Model file for the job. Use its own axes, mm. Round coordinates to 2 decimals unless told otherwise and drop trailing zeros. Write each loop counter-clockwise with the first axis right and the second up, starting at its lowest first coordinate (ties: lowest second). Pieces come first, ordered by that corner, then holes.
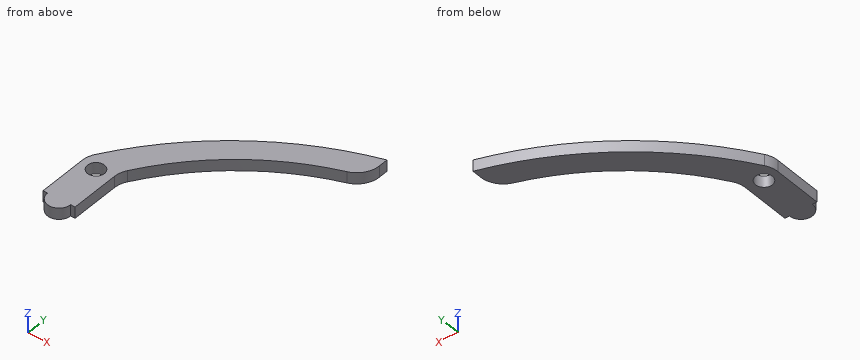
Autodesk Inventor part; units mm, degrees
ref_plane "YZ Plane" through (0, 0, 0) normal (1, 0, 0) x (0, 1, 0)
ref_plane "XZ Plane" through (0, 0, 0) normal (0, 1, 0) x (-1, 0, 0)
ref_plane "XY Plane" through (0, 0, 0) normal (0, 0, 1) x (1, 0, 0)
sketch "Sketch1" plane through (0, 0, 0) normal (0, 0, 1) x (1, 0, 0)
  circle A0 centre (-0.0549, 4.1489) radius 0.75
  line L0 (-1.4285, -0.0001) -> (-1.4285, 4.899)
  line L1 (-1.4285, 4.899) -> (1.4285, 4.899) construction
  line L2 (1.4285, 4.899) -> (1.4285, 0)
  circle A1 centre (0, 0) radius 1.0285
  line L3 (-1.0285, -0.0001) -> (-1.4285, -0.0001)
  line L4 (1.0285, 0) -> (1.4285, 0)
  line L5 (0, 0) -> (15, 0)
  arc A2 (15, 17.5757) -> (-1.4285, 4.899) centre (23.253, -10.1036) ccw
  arc A3 (15, 15.2472) -> (1.4285, 4.899) centre (21.0936, -6.818) ccw
  line L6 (15, 15.2472) -> (15, 17.5757)
  point P0 (0.0155, 4.8988)
  dimension "d6" = 1.5
  dimension "d28" = 2.057
  dimension "d29" = 0.4
  dimension "d30" = 0.4
  dimension "d33" = 15
extrude "Extrusion1" add sketch "Sketch1" along normal blind 1 contours L0 A2 L6 A3 L2 L4 A1 L3
extrude "Extrusion2" add sketch "Sketch1" along normal blind 1 contours A1
fillet "Fillet5" radius 2 3 edges at (15, 15.2472, 0.5) (-1.4285, 4.899, 0.5) (1.4285, 4.899, 0.5)
properties material "Nickel-Copper Alloy 400"
1) Cut at A-A on z = 0.75. List the corners of the cut face in (x, y).
2) Flat gauge pin, fed straight in: pin 1 Ø4 at (x, y) = (10, 9) entering from -Z. Where does the tip first touch, or does it go through?
3) Cut at D-D on x = 4. List the corners of the cut face in (y, z), and give its area (3 significant figures).
4) Cut at B-B on x = 0.25. List the corners of the cut face in (y, z).
5) Cut at C-C on y = 2.75. List the corners of the cut face in (x, z), and give its area (3 significant figures).
6) Wall check: probe 1 along Y at (x, z) = (-0.5, 0.15); probe 2 along Y at (x, z) = (-0.25, 0.7); probe 3 along X at (y, z) = (3, 0.45). Give the ranges that are in metal, low to high.
Result sheet:
1. outline: (-1.43, 0) - (-1.03, 0) arc R1.03 ccw to (1.03, 0) - (1.43, 0) - (1.43, 4.33) arc R2 cw to (1.74, 5.4) arc R22.89 cw to (13.65, 14.83) arc R2 ccw to (15, 16.72) - (15, 17.58) arc R28.88 ccw to (-1.12, 5.4) arc R2 ccw to (-1.43, 4.33) - close; hole circle Ø1.5 at (-0.05, 4.15)
2. pin 1: passes through
3. outline: (8.41, 0) - (11.43, 0) - (11.43, 1) - (8.41, 1) - close
3. area: 3.02 mm2
4. outline: (-1, 0) - (3.46, 0) - (3.46, 1) - (-1, 1) - close; (4.83, 0) - (7.36, 0) - (7.36, 1) - (4.83, 1) - close
5. outline: (-1.43, 0) - (1.43, 0) - (1.43, 1) - (-1.43, 1) - close
5. area: 2.86 mm2
6. probe 1: y = -0.9 to 3.55, 4.75 to 6.33
6. probe 2: y = -1 to 3.42, 4.87 to 6.69
6. probe 3: x = -1.43 to 1.43
